Geometry: final body of the model. Coordinates: model frame, mm. A direction names the side the tool comes from. Coordinates: 2 decimals unless noted, no trailing zeros. Write each loop counter-clockwise with the first axis right and the second up, starting at its lowest first coordinate (ties: lowest second). Pieces come first, ordered by that corner, then holes.
from build123d import *

# Parameters (mm, degrees)
SKETCH083_W   = 9
SKETCH083_H   = 64
PAD058_DEPTH  = 1
SKETCH084_W   = 9
SKETCH084_H   = 64
SKETCH084_W_2 = 7
SKETCH084_H_2 = 62
PAD059_DEPTH  = 3
BOX003_W      = 11
BOX003_H      = 66
BOX003_DEPTH  = 5


with BuildPart() as sidemold001:
    # Sketch083 → Pad058 (new body)
    with BuildSketch(Plane.XY):
        Rectangle(SKETCH083_W, SKETCH083_H)
    extrude(amount=PAD058_DEPTH)

    # Sketch084 (on Face6 of Pad058) → Pad059 (join)
    with BuildSketch(Plane.XY.offset(1)):
        Rectangle(SKETCH084_W, SKETCH084_H)
        Rectangle(SKETCH084_W_2, SKETCH084_H_2, mode=Mode.SUBTRACT)
    extrude(amount=PAD059_DEPTH)


with BuildPart() as sidemold001_1:
    # Body026 placement: moved
    add(sidemold001.part.moved(Location((150, 35, 0))))


with BuildPart() as long_side_mold:
    # Box003 → Box003 (new body)
    with BuildSketch(Plane(origin=(144.5, 2, 0), x_dir=(1, 0, 0), z_dir=(0, 0, 1))):
        with Locations((5.5, 33)):
            Rectangle(BOX003_W, BOX003_H)
    extrude(amount=BOX003_DEPTH)

    # Cut003: cut SideMold001
    add(sidemold001_1.part, mode=Mode.SUBTRACT)


with BuildPart() as long_side_mold_1:
    # Cut003 placement: moved
    add(long_side_mold.part.moved(Location((0, -19, 0))))


solid = long_side_mold_1.part
Item 1: Section B-B, the plane y = -8. Output: boundary loops of the cut face in (x, z), plus the area to 3 significant figures.
Derived:
outline: (144.5, 0) - (145.5, 0) - (145.5, 4) - (146.5, 4) - (146.5, 1) - (153.5, 1) - (153.5, 4) - (154.5, 4) - (154.5, 0) - (155.5, 0) - (155.5, 5) - (144.5, 5) - close
area: 40.0 mm2
Item 2: Material intervals for probe 1 along X at (y, z) = (36, 1.2); probe 2 along Y at (x, z) = (149.5, 1.4); probe 3 along Y at (x, z) = (152, 0.9), sorted ascending.
Derived:
probe 1: x = 144.5 to 145.5, 146.5 to 153.5, 154.5 to 155.5
probe 2: y = -17 to -16, -15 to 47, 48 to 49
probe 3: y = -17 to -16, 48 to 49
Item 3: Pin query (flat end, axial travel): pin 1 (2 mm diameter, centred on x = 150.5, y = 41, fed in from -Z). Return the tip coordinate at first contact, or that it passes through.
Derived:
pin 1: stops at z = 1
Item 4: Pull-direction query (Y, two-part tool) for faces 1 (the flat face through (150, -17, 2)), 2 (the flat face through (150, 48, 2)), 3 (the flat face through (154, 16, 4)), 4 (the flat face through (150, 16, 5)); classes: released by +Y, released by -Y, zero draft, split by the parting line, or undercut.
Derived:
face 1: released by -Y
face 2: undercut
face 3: undercut
face 4: zero draft
Item 5: Section A-A, the plane z = 1.9. Output: boundary loops of the cut face in (x, y), plus the area to 3 significant figures.
Derived:
outline: (144.5, -17) - (155.5, -17) - (155.5, 49) - (144.5, 49) - close; (146.5, -15) - (153.5, -15) - (153.5, 47) - (146.5, 47) - close; hole (145.5, -16) - (154.5, -16) - (154.5, 48) - (145.5, 48) - close
area: 584 mm2
Item 6: Section C-C, the plane x = 152.25. Output: boundary loops of the cut face in (y, z), plus the area to 3 significant figures.
Derived:
outline: (-17, 0) - (-16, 0) - (-16, 4) - (-15, 4) - (-15, 1) - (47, 1) - (47, 4) - (48, 4) - (48, 0) - (49, 0) - (49, 5) - (-17, 5) - close
area: 260 mm2
Item 7: Set-up query: faces 5 (the flat face through (145, 16, 0)), 6 (the flat face through (145.5, 16, 2)). Return all of +Z, -Z, +X, -X, +Y, -Y with unobstructed straight access to the full face (end or side cutting, diameter ignored); none if empty.
Derived:
face 5: -Z, +X, -X, +Y, -Y
face 6: -Z
